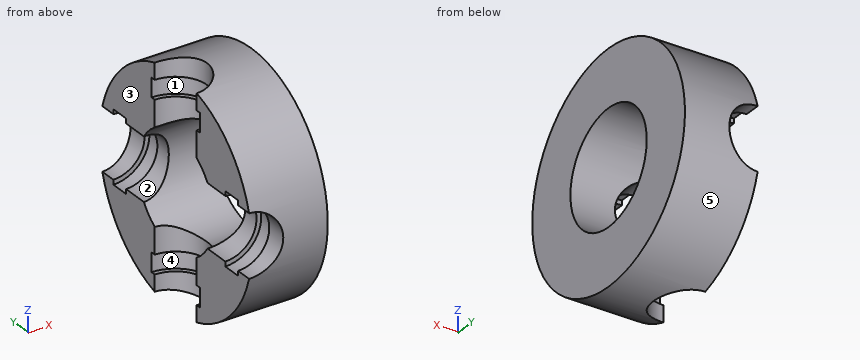
```python
from build123d import *

# Parameters (mm, degrees)
SKETCH1_R           = 30
SKETCH1_R_2         = 15
BOSS_EXTRUDE1_DEPTH = 40
SKETCH2_R           = 9.5
CUT_EXTRUDE1_DEPTH  = 2.5
SKETCH3_R           = 8.25
CUT_EXTRUDE2_DEPTH  = 15
CIRPATTERN1_COUNT   = 4


with BuildPart() as part:
    # Sketch1 → Boss-Extrude1 (new body)
    with BuildSketch(Plane(origin=(0, 0, 0), x_dir=(0, 0, -1), z_dir=(1, 0, 0))):
        Circle(SKETCH1_R)
        Circle(SKETCH1_R_2, mode=Mode.SUBTRACT)
    extrude(amount=BOSS_EXTRUDE1_DEPTH)

    # Sketch2 → Cut-Extrude1 (cut, symmetric)
    with BuildSketch(Plane.XY.offset(22)):
        with Locations((20, 0)):
            Circle(SKETCH2_R)
    cut_extrude1 = extrude(amount=CUT_EXTRUDE1_DEPTH, both=True, mode=Mode.SUBTRACT)

    # Sketch3 → Cut-Extrude2 (cut, symmetric)
    with BuildSketch(Plane.XY.offset(22)):
        with Locations((20, 0)):
            Circle(SKETCH3_R)
    cut_extrude2 = extrude(amount=CUT_EXTRUDE2_DEPTH, both=True, mode=Mode.SUBTRACT)

    # CirPattern1: Cut-Extrude1, Cut-Extrude2 ×4 about axis
    cirpattern1_axis = Axis((0, 0, 0), (1, 0, 0))
    for i in range(1, CIRPATTERN1_COUNT):
        add(cut_extrude1.rotate(cirpattern1_axis, i * 360 / CIRPATTERN1_COUNT), mode=Mode.SUBTRACT)
        add(cut_extrude2.rotate(cirpattern1_axis, i * 360 / CIRPATTERN1_COUNT), mode=Mode.SUBTRACT)


with BuildPart() as body_2:
    # Split2: the piece on the far side of the plane
    add(part.part)
    split(bisect_by=Plane(origin=(20, 0, 0), x_dir=(0, 0, 1), z_dir=(1, 0, 0)), keep=Keep.BOTTOM)


with BuildPart() as part_1:
    add(part.part)

    # Split2
    split(bisect_by=Plane(origin=(20, 0, 0), x_dir=(0, 0, 1), z_dir=(1, 0, 0)), keep=Keep.TOP)


solid = part_1.part
```
Read the model definition and answer for the solid it produces. Units are mm, in the model's axes. Face numbers are marked on the shaded views. A direction names the side the tool comes from. Coordinates: 2 decimals unless noted, no trailing zeros. Write each loop counter-clockwise with the first axis right and the second up, starting at its lowest first coordinate (ties: lowest second). Pieces come first, ordered by that corner, then holes. Notation, with made-up numbers: (40.25, 31) -> (68.25, 31) arc R14 ccw to (68.25, 44) -> close; hole circle Ø6 at (23, -28). An arc over 180 degrees is marked (long way). Return JSON: item names as keys, results as strings.
1. A cutting plane is placed at A-A (z = 0). Determine the outline of the cut face in (x, y).
Found:
{"outline": "(28.25, -30) -> (40, -30) -> (40, -15) -> (28.25, -15) -> (28.25, -19.5) -> (29.5, -19.5) -> (29.5, -24.5) -> (28.25, -24.5) -> close; (28.25, 15) -> (40, 15) -> (40, 30) -> (28.25, 30) -> (28.25, 24.5) -> (29.5, 24.5) -> (29.5, 19.5) -> (28.25, 19.5) -> close"}
2. A cutting plane is placed at B-B (y = 3.5). Determine the outline of the cut face in (x, z).
Found:
{"outline": "(27.47, -29.8) -> (40, -29.8) -> (40, -14.59) -> (27.47, -14.59) -> (27.47, -19.5) -> (28.83, -19.5) -> (28.83, -24.5) -> (27.47, -24.5) -> close; (27.47, 14.59) -> (40, 14.59) -> (40, 29.8) -> (27.47, 29.8) -> (27.47, 24.5) -> (28.83, 24.5) -> (28.83, 19.5) -> (27.47, 19.5) -> close"}
3. A cutting plane is placed at C-C (x = 37). Determine the outline of the cut face in (y, z), and give its area (3 significant figures).
Found:
{"outline": "circle Ø60 at (0, 0); hole circle Ø30 at (0, 0)", "area": "2,120 mm2"}
4. Determine the mould class of the marked faces 3, 4 and 5 for opening direction Y: pulls with the +Y half, pulls with the -Y half, needs draft (parallel to the pull), parting line crosses it, or undercut.
Found:
{"face 3": "needs draft", "face 4": "undercut", "face 5": "parting line crosses it"}
5. A cutting plane is placed at D-D (z = 13.5). Determine the outline of the cut face in (x, y), and give its area (3 significant figures).
Found:
{"outline": "(20, -26.79) -> (40, -26.79) -> (40, -6.54) -> (25.03, -6.54) arc R8.25 cw to (20, -8.25) -> close; (20, 8.25) arc R8.25 cw to (25.03, 6.54) -> (40, 6.54) -> (40, 26.79) -> (20, 26.79) -> close", "area": "798 mm2"}
6. A tool of negligible diameter and unlimited length cuts with its end or side. For the marked faces 1 and 2, from which of +Z, -Z, +X, -X, +Y, -Y can it reach the whole face along a straight path? Write none if from no direction.
Found:
{"face 1": "-X", "face 2": "-X, +Y, -Y"}
7. Each of these flat-tipped pins is pushed along its axis until it touches: P1, Ø10, axis at x = 33, y = -20, coming from the +Z side; P2, Ø1.5, axis at x = 25.5, y = 10, coming from the -Z side; P3, Ø8, axis at y = 18, z = 0, coming from the -X side. Where does it stop, or does it pass through?
Found:
{"P1": "z = 25.98", "P2": "z = -28.54", "P3": "x = 27.22"}
8. Find the intervals of material crossed by line 1 along Y through (x, z) = (29, 0); line 2 along Y through (x, z) = (22.75, -11); line 3 along Z through (x, y) = (31.75, 2.5), in increasing order. Write a range as from..to.
Found:
{"line 1": "-30..-24.5, -19.5..-15, 15..19.5, 24.5..30", "line 2": "-27.91..-10.2, 10.2..27.91", "line 3": "-29.9..-14.79, 14.79..29.9"}
